Autodesk Inventor part; units mm, degrees
ref_plane "YZ Plane" through (0, 0, 0) normal (1, 0, 0) x (0, 1, 0)
ref_plane "XZ Plane" through (0, 0, 0) normal (0, 1, 0) x (-1, 0, 0)
ref_plane "XY Plane" through (0, 0, 0) normal (0, 0, 1) x (1, 0, 0)
sketch "Sketch1" plane through (0, 0, 0) normal (0, 1, 0) x (-1, 0, 0)
  line L0 (3.175, 0) -> (9.525, 0)
  line L1 (12.7, 3.175) -> (12.7, 98.425)
  line L2 (9.525, 101.6) -> (3.175, 101.6)
  line L3 (0, 98.425) -> (0, 3.175)
  circle A0 centre (6.35, 95.25) radius 2.5797
  circle A1 centre (6.35, 6.35) radius 2.5797
  arc A2 (12.7, 98.425) -> (9.525, 101.6) centre (9.525, 98.425) ccw
  arc A3 (3.175, 101.6) -> (0, 98.425) centre (3.175, 98.425) ccw
  arc A4 (0, 3.175) -> (3.175, 0) centre (3.175, 3.175) ccw
  arc A5 (9.525, 0) -> (12.7, 3.175) centre (9.525, 3.175) ccw
  point P0 (0, 0)
  point P1 (12.7, 101.6)
  point P2 (0, 101.6)
  dimension "d0" = 12.7
  dimension "d1" = 101.6
  dimension "d2" = 6.35
  dimension "d3" = 6.35
  dimension "d4" = 6.35
  dimension "d5" = 6.35
  dimension "d6" = 5.1594
  dimension "d7" = 3.175
extrude "Extrusion1" add sketch "Sketch1" along normal blind 3.175
equation "\"d2\" = 0.5 * d0"
equation "\"d3\" = d2"
equation "\"d4\" = d3"
equation "\"d5\" = d4"
properties part number "Pusher"
Build history of the part. All positions in model axes, mm. Give positions to 0.01 mm unless a question says otherwise; leave off trailing zeros. Loops run counter-clockwise (first coordinate to the right, second up) from the corner with the lowest first, then second, coordinate; pieces in that order, holes last. Notation, with made-up numbers: (-28, 55.5) -> (3, 55.5) arc R21 ccw to (3, 87.5) -> close; hole circle Ø2 at (-22, 88.5). An arc over 180 degrees is marked (long way). One line per question, with ' | ' between items. Start each with the question number.
1) Two-plate mould, pull along X, no slides. Class faces 1 (the flat face through (-12.7, 2, 50)), 2 (the cylindrical face through (-0.91, 1.57, 100.65)), 3 (the cylindrical face through (-7.54, 1.57, 97.54)): released by +X, released by -X, zero draft, split by the parting line, or undercut.
2) Cut at B-B (y = 1.1). Give the cut face in (x, z) (3 decimals).
3) Cut at C-C (x = -6.35). Give the cut face in (y, z) (3 decimals).
4) Probe L1, parallel to Z at x = -6.35, y = 1.9; L2, parallel to Z at x = -4.25, y = 2.8; L3, parallel to X at y = 2, z = 95.5. List the from-to ranges inside material, lowest first.
5) Cut at A-A (z = 95.25). Give the cut face in (x, y) (3 decimals), plus the area to 3 significant figures.
6) Pin check, flat tips, straight feed: pin 1 (3 mm diameter, centred on x = -10.5, z = 13, fed in from -Y); pin 2 (4 mm diameter, centred on x = -6.35, z = 95.25, fed in from -Y). Stop position of each tip, or through.
Return value:
1) face 1: released by -X | face 2: released by +X | face 3: undercut
2) outline: (-12.7, 3.175) arc R3.175 ccw to (-9.525, 0) -> (-3.175, 0) arc R3.175 ccw to (0, 3.175) -> (0, 98.425) arc R3.175 ccw to (-3.175, 101.6) -> (-9.525, 101.6) arc R3.175 ccw to (-12.7, 98.425) -> close; hole circle Ø5.159 at (-6.35, 6.35); hole circle Ø5.159 at (-6.35, 95.25)
3) outline: (0, 0) -> (3.175, 0) -> (3.175, 3.77) -> (0, 3.77) -> close; (0, 8.93) -> (3.175, 8.93) -> (3.175, 92.67) -> (0, 92.67) -> close; (0, 97.83) -> (3.175, 97.83) -> (3.175, 101.6) -> (0, 101.6) -> close
4) L1: 0 to 3.77, 8.93 to 92.67, 97.83 to 101.6 | L2: 0 to 4.85, 7.85 to 93.75, 96.75 to 101.6 | L3: -12.7 to -8.92, -3.78 to 0
5) outline: (-12.7, 0) -> (-8.93, 0) -> (-8.93, 3.175) -> (-12.7, 3.175) -> close; (-3.77, 0) -> (0, 0) -> (0, 3.175) -> (-3.77, 3.175) -> close | area: 23.9 mm^2
6) pin 1: y = 0 | pin 2: through
